from build123d import *

# Parameters (mm, degrees)
F17_DEPTH = 7.5
F19_DEPTH = 7.5
F20_DEPTH = 7.5


# Not quite as in the source:
# - the arcs of a loft's sections are written as splines that run evenly, so that the points pair up as in the source's solid


with BuildPart() as f9:
    # F2 (on face) → F9 section 0
    with BuildSketch(Plane(origin=(5, -5, 0), x_dir=(0.7071067812, 0.7071067812, 0), z_dir=(0.7071067812, -0.7071067812, 0))):
        with BuildLine():
            add(Edge.make_bspline(
                [(53.6396103068, 0), (53.6396103068, -0.5817764173), (53.7421679492, -1.1634097103), (54.1401264565, -2.2567917229), (54.4354294185, -2.7682714568), (55.1833467639, -3.6596046401), (55.6357771501, -4.0392388103), (56.1396103068, -4.3301270189)],
                knots=[0, 0, 0, 0, 0.3333333333, 0.3333333333, 0.6666666667, 0.6666666667, 1, 1, 1, 1], degree=3))
            add(Edge.make_bspline(
                [(56.1396103068, -4.3301270189), (56.6434434635, -4.6210152276), (57.1984314921, -4.8230143504), (58.3443073448, -5.0250631797), (58.9349132688, -5.0250631797), (60.0807891214, -4.8230143504), (60.6357771501, -4.6210152276), (61.1396103068, -4.3301270189)],
                knots=[0, 0, 0, 0, 0.3333333333, 0.3333333333, 0.6666666667, 0.6666666667, 1, 1, 1, 1], degree=3))
            add(Edge.make_bspline(
                [(61.1396103068, -4.3301270189), (61.6434434635, -4.0392388103), (62.0958738497, -3.6596046401), (62.8437911951, -2.7682714568), (63.1390941571, -2.2567917229), (63.5370526644, -1.1634097103), (63.6396103068, -0.5817764173), (63.6396103068, 0)],
                knots=[0, 0, 0, 0, 0.3333333333, 0.3333333333, 0.6666666667, 0.6666666667, 1, 1, 1, 1], degree=3))
            add(Edge.make_bspline(
                [(63.6396103068, 0), (63.6396103068, 0.5817764173), (63.5370526644, 1.1634097103), (63.1390941571, 2.2567917229), (62.8437911951, 2.7682714568), (62.0958738497, 3.6596046401), (61.6434434635, 4.0392388103), (61.1396103068, 4.3301270189)],
                knots=[0, 0, 0, 0, 0.3333333333, 0.3333333333, 0.6666666667, 0.6666666667, 1, 1, 1, 1], degree=3))
            add(Edge.make_bspline(
                [(61.1396103068, 4.3301270189), (60.6357771501, 4.6210152276), (60.0807891214, 4.8230143504), (58.9349132688, 5.0250631797), (58.3443073448, 5.0250631797), (57.1984314921, 4.8230143504), (56.6434434635, 4.6210152276), (56.1396103068, 4.3301270189)],
                knots=[0, 0, 0, 0, 0.3333333333, 0.3333333333, 0.6666666667, 0.6666666667, 1, 1, 1, 1], degree=3))
            add(Edge.make_bspline(
                [(56.1396103068, 4.3301270189), (55.6357771501, 4.0392388103), (55.1833467639, 3.6596046401), (54.4354294185, 2.7682714568), (54.1401264565, 2.2567917229), (53.7421679492, 1.1634097103), (53.6396103068, 0.5817764173), (53.6396103068, 0)],
                knots=[0, 0, 0, 0, 0.3333333333, 0.3333333333, 0.6666666667, 0.6666666667, 1, 1, 1, 1], degree=3))
        make_face()
    # F8 (on plane+point) → F9 section 1
    with BuildSketch(Plane.XZ.offset(-26.335299015)):
        Polygon((38.9644660941, 7.5), (38.9644660941, 0), (38.9644660941, -7.5), (53.9644660941, -7.5), (53.9644660941, 0), (53.9644660941, 7.5), align=None)
    loft(ruled=True)

    # F16 (on plane+point) → F17 (join, symmetric)
    with BuildSketch(Plane.XY):
        with BuildLine():
            ThreePointArc((38.9644660941, 26.335299015), (34.8752223254, 23.4990929499), (30, 22.5))
            Line((30, 22.5), (30, 7.5))
            ThreePointArc((30, 7.5), (45.2402766064, 12.7723861725), (53.9644660941, 26.335299015))
            Line((53.9644660941, 26.335299015), (38.9644660941, 26.335299015))
        make_face()
    extrude(amount=F17_DEPTH, both=True)

    # F18 (on Top) → F19 (join, symmetric)
    with BuildSketch(Plane.XY):
        Polygon((30, 7.5), (30, 22.5), (25, 22.5), (25, 15), (25, 7.5), align=None)
    extrude(amount=F19_DEPTH, both=True)

    # F18 (on Top) → F20 (join, symmetric)
    with BuildSketch(Plane.XY):
        with BuildLine():
            Line((-50, 40), (-20, 40))
            ThreePointArc((-20, 40), (-34.1886116992, 47.4341649025), (-50, 50))
            Line((-50, 50), (-50, 40))
        make_face()
        with BuildLine():
            Line((25, 15), (25, 22.5))
            ThreePointArc((25, 22.5), (4.5562384252, 26.3545057073), (-14.0947561264, 35.5710670948))
            ThreePointArc((-14.0947561264, 35.5710670948), (-17.1007926042, 37.7143141594), (-20, 40))
            Line((-20, 40), (-50, 40))
            Line((-50, 40), (-50, 30))
            ThreePointArc((-50, 30), (-34.1886116992, 27.4341649025), (-20, 20))
            ThreePointArc((-20, 20), (-18.1598300563, 17.7950849719), (-17.5, 15))
            Line((-17.5, 15), (10, 15))
            Line((10, 15), (25, 15))
        make_face()
        with BuildLine():
            ThreePointArc((-20, -43.971782705), (8.4686762609, -23.4540986425), (25, 7.5))
            ThreePointArc((25, 7.5), (18.3458720417, 6.87456335), (11.7716580953, 5.6711096222))
            ThreePointArc((11.7716580953, 5.6711096222), (-13.5991721952, -22.4348243888), (-50, -32.8560667038))
            Line((-50, -32.8560667038), (-50, -42.8560667038))
            Line((-50, -42.8560667038), (-50, -50))
            ThreePointArc((-50, -50), (-34.7001682709, -48.4780326329), (-20, -43.971782705))
        make_face()
        with BuildLine():
            Line((25, 7.5), (25, 15))
            Line((25, 15), (10, 15))
            Line((10, 15), (11.7716580953, 5.6711096222))
            ThreePointArc((11.7716580953, 5.6711096222), (18.3458720417, 6.87456335), (25, 7.5))
        make_face()
        with BuildLine():
            Line((11.7716580953, 5.6711096222), (10, 15))
            Line((10, 15), (-17.5, 15))
            ThreePointArc((-17.5, 15), (-18.1598300563, 12.2049150281), (-20, 10))
            ThreePointArc((-20, 10), (-34.1886116992, 2.5658350975), (-50, 0))
            Line((-50, 0), (-50, -20))
            ThreePointArc((-50, -20), (-34.1886116992, -17.4341649025), (-20, -10))
            ThreePointArc((-20, -10), (-19.4528820076, -9.5510950315), (-18.9016373284, -9.1072672811))
            ThreePointArc((-18.9016373284, -9.1072672811), (-4.3970359749, 0.0088769739), (11.7716580953, 5.6711096222))
        make_face()
    extrude(amount=F20_DEPTH, both=True)


solid = f9.part
Verification items for the finished model (mm, model axes). A direction names the side the tool comes from. Give positions to 0.01 mm unless a question says otherwise; leave off trailing zeros. Loops run counter-clockwise (first coordinate to the right, second up) from the corner with the lowest first, then second, coordinate; pieces in that order, holes last. Notation, with made-up numbers: (73, 33.5) - (83, 33.5) arc R20 ccw to (83, 59.5) - close; hole circle Ø1 at (44, 12.25). An arc over 180 degrees is marked (long way). Write item = value, one per line. Start each with the question number.
Q1. Tool access check on faces 4 (the face through (-34.402, -17.505, 0.105)), 5 (the face through (46, 36, 0)), 6 (the face through (-34.402, 27.505, 0.105)), 7 (the face through (-33.975, 47.362, 0.105)), 8 (the face through (27, 7.5, 0)). Record the directions out of +Z, -Z, +X, -X, +Y, -Y that give a thin tool (end or side, any length) a straight path to the whole face; none if there is none.
Q2. Cross-section at C-C, the plane x = 27. Enter the section's corners in (y, z), and give its area (3 significant figures).
Q3. Thickness scan on line 1 (Y direction, x = -25.5, z = 0.75); line 2 (Y direction, x = -39.5, z = -3); line 3 (Y direction, x = 0.5, z = 3.5). Record the ranges inside material, lowest first.
Q4. Cross-section at D-D, the plane y = -29. Enter the section's corners in (x, z).
Q5. Mould release check, pull along Y, two halves, no side actions. Record for faces 1 (the face through (28, 22.5, 0)), 2 (the face through (-13.145, -22.149, 0.105)), 3 (the face through (-50, 40, 0)): released by +Y, released by -Y, zero draft, split by the parting line, or undercut.
Q6. Cross-section at B-B, the plane y = -4. Enter the section's corners in (x, z), and give its area (3 significant figures).
Q7. Cross-section at A-A, the plane x = -4. Enter the section's corners in (y, z), and give its area (3 significant figures).
Q8. Depth check by flat-ended pin: P1, Ø4, axis at y = -27, z = 0, coming from the +X side; P2, Ø8, axis at x = -31, z = -2, coming from the +Y side; P3, Ø4, axis at x = 28.5, z = 0, coming from the -Y side. Enter the tip coordinate at first touch or a pass-through.
Answer key:
q1.face_4 = +Z, -Z
q1.face_5 = +Z, -Z, +Y
q1.face_6 = +Z, -Z, -X
q1.face_7 = +Z, -Z, +X, +Y
q1.face_8 = +Z, -Z, +X, -Y
q2.outline = (7.5, -7.5) - (22.5, -7.5) - (22.5, 7.5) - (7.5, 7.5) - close
q2.area = 225 mm^2
q3.line_1 = -46.03 to -28.34, -13.59 to 6.41, 23.59 to 43.59
q3.line_2 = -49.29 to -32.05, -18.89 to 1.11, 28.89 to 48.89
q3.line_3 = -31.34 to -10.77, 2.16 to 27.84
q4.outline = (-27.29, -7.5) - (3.11, -7.5) - (3.11, 7.5) - (-27.29, 7.5) - close
q5.face_1 = released by +Y
q5.face_2 = undercut
q5.face_3 = zero draft
q6.outline = (-50, -7.5) - (-11.68, -7.5) - (-11.68, 7.5) - (-50, 7.5) - close; (6.01, -7.5) - (20.92, -7.5) - (20.92, 7.5) - (6.01, 7.5) - close
q6.area = 798 mm^2
q7.outline = (-34.91, -7.5) - (-15.21, -7.5) - (-15.21, 7.5) - (-34.91, 7.5) - close; (0.2, -7.5) - (29.8, -7.5) - (29.8, 7.5) - (0.2, 7.5) - close
q7.area = 740 mm^2
q8.P1 = 7.08
q8.P2 = 47.7
q8.P3 = 7.5
